Model file for the job. Use its own axes, mm. Face numbers are marked on the shaded views. Coordinates: 2 decimals unless noted, no trailing zeros. Write each loop counter-clockwise with the first axis right and the second up, starting at its lowest first coordinate (ties: lowest second). Pieces come first, ordered by that corner, then holes. Notation, with made-up numbers: (-2, 51.5) - (46, 51.5) arc R21 ccw to (46, 70.5) - close; hole circle Ø10 at (-11, -14). An arc over 180 degrees is marked (long way). Put each result on its own line as item: value. Start each with the question number.
1. Saw through at A-A, the plane y = 0. Write the cut outline in (x, z), plus the area to 3 significant figures.
2. Drill centre lines: L1, parallel to Y at x = 0, z = 3.75; L2, parallel to Y at x = 0, z = -23.5; L3, parallel to Z at x = 5.75, y = -4.5. Where is each one in solid material? Low to high. Write a range as from..to.
3. Saw through at C-C, the plane z = -20. Write the cut outline in (x, y), plus the area to 3 significant figures.
4. Pull direction Y, two halves, no side cores. Call the marked faces 1, 2 and 3: released by +Y, released by -Y, zero draft, split by the parting line, or undercut.
5. Drop flat-ended pins along their axis: P1, Ø8, axis at x = -2.5, y = 0, coming from the +Z side; P2, Ø6, axis at x = 4.5, z = -6.5, coming from the -Y side; P3, Ø8.5, axis at x = -0.5, y = 0.5, coming from the +Z side; P4, Ø2, axis at y = 2.5, z = -29, coming from the +X side. Give the stop position or say it passes through.
6. Saw through at D-D, the plane y = -3.75. Write the cut outline in (x, z), plus the area to 3 significant figures.
```python
from build123d import *

# Parameters (mm, degrees)
SKETCH1_R           = 7.7
SKETCH1_R_2         = 3.25
BOSS_EXTRUDE1_DEPTH = 5.85
SKETCH2_R           = 5.25
CUT_EXTRUDE1_DEPTH  = 1.2
SKETCH4_R           = 6
SKETCH4_R_2         = 3.25
BOSS_EXTRUDE2_DEPTH = 7
SKETCH5_R           = 6
SKETCH5_R_2         = 4.6
BOSS_EXTRUDE5_DEPTH = 30


with BuildPart() as part:
    # Sketch1 → Boss-Extrude1 (new body)
    with BuildSketch(Plane.XY):
        Circle(SKETCH1_R)
        Circle(SKETCH1_R_2, mode=Mode.SUBTRACT)
    extrude(amount=BOSS_EXTRUDE1_DEPTH)

    # Sketch2 → Cut-Extrude1 (cut)
    with BuildSketch(Plane.XY.offset(5.85)):
        Circle(SKETCH2_R)
    extrude(amount=-CUT_EXTRUDE1_DEPTH, mode=Mode.SUBTRACT)

    # Sketch4 → Boss-Extrude2 (add)
    with BuildSketch(Plane(origin=(0, 0, 0), x_dir=(-1, 0, 0), z_dir=(0, 0, -1))):
        Circle(SKETCH4_R)
        Circle(SKETCH4_R_2, mode=Mode.SUBTRACT)
    extrude(amount=BOSS_EXTRUDE2_DEPTH)

    # Sketch5 → Boss-Extrude5 (add)
    with BuildSketch(Plane(origin=(0, 0, -7), x_dir=(-1, 0, 0), z_dir=(0, 0, -1))):
        Circle(SKETCH5_R)
        Circle(SKETCH5_R_2, mode=Mode.SUBTRACT)
    extrude(amount=BOSS_EXTRUDE5_DEPTH)


solid = part.part
```
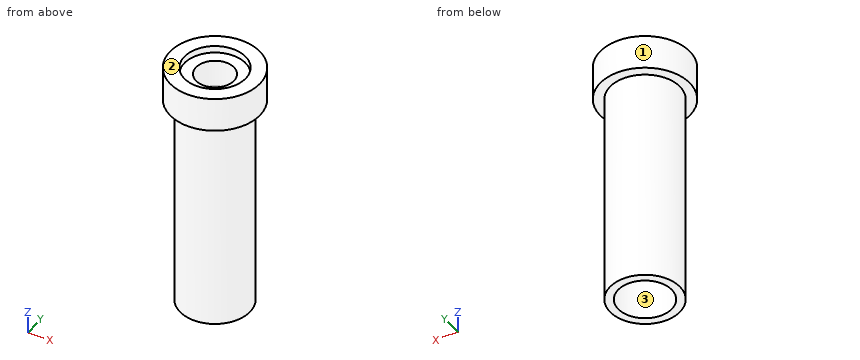
Final values:
1. outline: (-7.7, 0) - (-6, 0) - (-6, -37) - (-4.6, -37) - (-4.6, -7) - (-3.25, -7) - (-3.25, 4.65) - (-5.25, 4.65) - (-5.25, 5.85) - (-7.7, 5.85) - close; (3.25, -7) - (4.6, -7) - (4.6, -37) - (6, -37) - (6, 0) - (7.7, 0) - (7.7, 5.85) - (5.25, 5.85) - (5.25, 4.65) - (3.25, 4.65) - close
1. area: 170 mm²
2. L1: y = -7.7..-3.25, 3.25..7.7
2. L2: y = -6..-4.6, 4.6..6
2. L3: z = 0..5.85
3. outline: circle Ø12 at (0, 0); hole circle Ø9.2 at (0, 0)
3. area: 46.6 mm²
4. face 1: split by the parting line
4. face 2: zero draft
4. face 3: undercut
5. P1: stops at z = 5.85
5. P2: stops at y = -5.81
5. P3: stops at z = 4.65
5. P4: stops at x = 5.81
6. outline: (-6.73, 0) - (-4.68, 0) - (-4.68, -37) - (-2.66, -37) - (-2.66, -7) - (2.66, -7) - (2.66, -37) - (4.68, -37) - (4.68, 0) - (6.73, 0) - (6.73, 5.85) - (3.67, 5.85) - (3.67, 4.65) - (-3.67, 4.65) - (-3.67, 5.85) - (-6.73, 5.85) - close
6. area: 257 mm²
